The listing builds one solid part. Answer for the finished solid, in the listing's coordinates (mm). Coordinates: 2 decimals unless noted, no trailing zeros. Write each loop counter-clockwise with the first axis right and the second up, starting at its lowest first coordinate (ties: lowest second). Pieces come first, ordered by that corner, then holes. Notation, with made-up numbers: M 78.25,28.5 L 84.25,28.5 A22 cw 84.25,49.5 Z; hole C -19.5,-40 d10. An arc over 180 degrees is marked long. Write item = value, one per line. Start each with the question number.
```python
from build123d import *

# Parameters (mm, degrees)
EXTRUDE_1_DEPTH               = 30
SKETCH_5_R                    = 2.75
CUT_EXTRUDE_1_DEPTH           = 1
HOLE_WIZARD_M2_52_D           = 2.9
HOLE_WIZARD_M2_52_CSINK_D     = 5.5
HOLE_WIZARD_M2_52_CSINK_ANGLE = 90


with BuildPart() as part:
    # Эскиз1 → Бобышка-Вытянуть1 (new, symmetric)
    with BuildSketch(Plane.XY):
        Polygon((-10, -3), (-10, 3), (-6, 3), (-3, 7.5), (0, 7.5), (0, -7.5), (-3, -7.5), (-6, -3), align=None)
    extrude(amount=EXTRUDE_1_DEPTH, both=True)

    # Эскиз5 → Вырез-Вытянуть1 (cut)
    with BuildSketch(Plane(origin=(0, 0, 0), x_dir=(0, 0, -1), z_dir=(1, 0, 0))):
        with Locations((-24, 0)):
            Circle(SKETCH_5_R)
        with Locations((24, 0)):
            Circle(SKETCH_5_R)
    extrude(amount=-CUT_EXTRUDE_1_DEPTH, mode=Mode.SUBTRACT)

    # Зенковка для винта с потайной головкой M2.52 (through all)
    with Locations(Plane(origin=(-1, 0, 0), x_dir=(0, 0, -1), z_dir=(1, 0, 0))):
        with Locations((-24, 0), (24, 0)):
            CounterSinkHole(HOLE_WIZARD_M2_52_D / 2, HOLE_WIZARD_M2_52_CSINK_D / 2, counter_sink_angle=HOLE_WIZARD_M2_52_CSINK_ANGLE)


solid = part.part
```
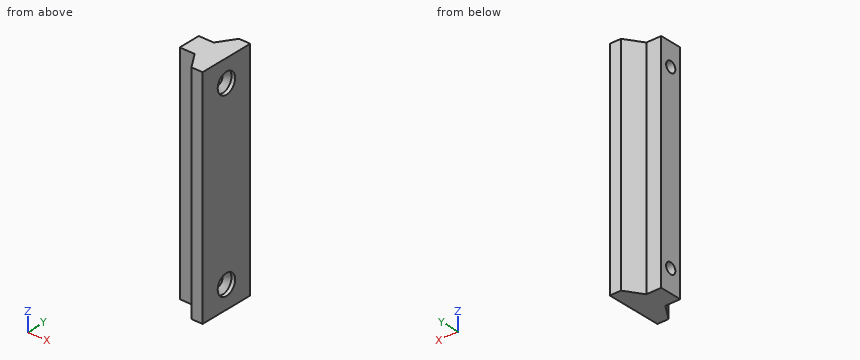
1. The part is cut by section B-B, the plane y = 0. Write down the section's boundary in (x, z).
2. The part is cut by section A-A, the plane z = 24. Write down the section's boundary in (x, y).
3. The part is cut by section C-C, the plane x = -7.25. Write down the section's boundary in (y, z), and give its area (3 significant figures).
4. Straight lines are drawn through the part: L1, parallel to Z at x = -5.75, y = 0; L2, parallel to Z at x = -0.35, y = 0; L3, parallel to Y at x = -7, z = 24. For each, find the intervals that lie inside material, in ascending order. Write a range as [from, to].
5. The part is cut by section D-D, the plane z = -6. Write down the section's boundary in (x, y), and give its area (4 significant figures).
6. Each of these flat-tipped pins is pushed along its axis until it touches: pin 1 (1.2 mm diameter, centred on x = -8.5, z = 8.5, fed in from -Y); pin 2 (2 mm diameter, centred on y = -5, z = -13, fed in from -X); pin 3 (6 mm diameter, centred on x = -8.5, z = -10, fed in from -Y). Where does it stop, or does it pass through?
Solution:
q1.outline = M -10,-30 L 0,-30 L 0,-26.75 L -1,-26.75 L -2.3,-25.45 L -10,-25.45 Z; M -10,-22.55 L -2.3,-22.55 L -1,-21.25 L 0,-21.25 L 0,21.25 L -1,21.25 L -2.3,22.55 L -10,22.55 Z; M -10,25.45 L -2.3,25.45 L -1,26.75 L 0,26.75 L 0,30 L -10,30 Z
q2.outline = M -10,-3 L -6,-3 L -3,-7.5 L 0,-7.5 L 0,-2.75 L -1,-2.75 L -2.3,-1.45 L -10,-1.45 Z; M -10,1.45 L -2.3,1.45 L -1,2.75 L 0,2.75 L 0,7.5 L -3,7.5 L -6,3 L -10,3 Z
q3.outline = M -3,-30 L 3,-30 L 3,30 L -3,30 Z; hole C 0,-24 d2.9; hole C 0,24 d2.9
q3.area = 347 mm^2
q4.L1 = [-30, -25.45], [-22.55, 22.55], [25.45, 30]
q4.L2 = [-30, -26.75], [-21.25, 21.25], [26.75, 30]
q4.L3 = [-3, -1.45], [1.45, 3]
q5.outline = M -10,-3 L -6,-3 L -3,-7.5 L 0,-7.5 L 0,7.5 L -3,7.5 L -6,3 L -10,3 Z
q5.area = 100.5 mm^2
q6.pin_1 = -3
q6.pin_2 = -5.33
q6.pin_3 = -3.75
